Source: CAD feature listing. Evaluate the final solid. Frame: model axes, mm. A direction names the side the tool comes from. Coordinates: 2 decimals unless noted, no trailing zeros. Order: outer loops, then holes, each group sorted by start corner. A loop starts at its lowest first (then second) coordinate and runs counter-clockwise, first axis right, second up.
Autodesk Inventor part; units mm, degrees
ref_plane "YZ Plane" through (0, 0, 0) normal (1, 0, 0) x (0, 1, 0)
ref_plane "XZ Plane" through (0, 0, 0) normal (0, 1, 0) x (-1, 0, 0)
ref_plane "XY Plane" through (0, 0, 0) normal (0, 0, 1) x (1, 0, 0)
sketch "Sketch1" plane through (0, 0, 0) normal (0, 1, 0) x (-1, 0, 0)
  line L0 (10, -14) -> (-10, -14)
  line L1 (-10, -14) -> (-10, 14)
  line L2 (-10, 14) -> (10, 14)
  line L3 (10, 14) -> (10, -14)
  line L4 (10, -14) -> (-10, 14) construction
  line L5 (-10, -14) -> (10, 14) construction
  point P0 (0, 0)
  dimension "d0" = 20
  dimension "d1" = 28
extrude "Extrusion1" add sketch "Sketch1" along normal blind 3
sketch "Sketch2" plane through (0, 0, 0) normal (0, -1, 0) x (1, 0, 0)
  line L0 (-10, 14) -> (10, 14)
  line L1 (-10, 14) -> (10, 14)
  line L2 (10, 14) -> (10, 11)
  line L3 (10, 11) -> (-10, 11)
  line L4 (-10, 11) -> (-10, 14)
  point P0 (0, 0)
  dimension "d4" = 20
  dimension "d5" = 3
extrude "Extrusion2" add sketch "Sketch2" along normal blind 25
sketch "Sketch3" plane through (10, 0, -14) normal (1, 0, 0) x (0, 0, -1)
  line L0 (-25, 0) -> (-25, -25)
  line L1 (0, 0) -> (-25, 0)
  line L2 (0, 0) -> (-25, 0)
  line L3 (-25, 0) -> (-25, -25)
  line L4 (-25, -25) -> (-22, -25)
  line L5 (-22, -25) -> (-22, -22)
  line L6 (0, 0) -> (0, 3)
  line L7 (0, 0) -> (0, -3)
  line L8 (0, -3) -> (-3, -3)
  line L9 (-3, -3) -> (-22, -22)
  point P0 (-14, 0)
  dimension "d8" = 3
  dimension "d9" = 3
  dimension "d10" = 3
  dimension "d11" = 3
extrude "Extrusion3" add sketch "Sketch3" against normal blind 2
mirror "Mirror1" about plane through (0, 0, 0) normal (1, 0, 0) of "Extrusion3"
sketch "Sketch4" plane through (-10, 3, 14) normal (0, 0, 1) x (1, 0, 0)
  line L0 (2, -28) -> (18, -28)
  line L1 (6.75, -9) -> (13.25, -9)
  line L2 (13.25, -9) -> (13.25, -19)
  line L3 (13.25, -19) -> (6.75, -19)
  line L4 (6.75, -19) -> (6.75, -9)
  line L5 (6.75, -9) -> (13.25, -19) construction
  line L6 (13.25, -9) -> (6.75, -19) construction
  arc A0 (13.25, -9) -> (6.75, -9) centre (10, -9) ccw
  arc A1 (6.75, -19) -> (13.25, -19) centre (10, -19) ccw
  point P0 (10, -3)
  point P1 (10, -14)
  dimension "d14" = 6.5
  dimension "d15" = 10
extrude "Extrusion4" cut sketch "Sketch4" against normal through all
sketch "Sketch5" plane through (0, 3, 0) normal (0, 1, 0) x (1, 0, 0)
  line L0 (3.25, -5) -> (-3.25, -5)
  line L1 (-3.25, -5) -> (-3.25, 5)
  line L2 (-3.25, 5) -> (3.25, 5)
  line L3 (3.25, 5) -> (3.25, -5)
  line L4 (3.25, -5) -> (-3.25, 5) construction
  line L5 (-3.25, -5) -> (3.25, 5) construction
  arc A0 (-3.25, -5) -> (3.25, -5) centre (0, -5) ccw
  arc A1 (3.25, 5) -> (-3.25, 5) centre (0, 5) ccw
  point P0 (0, 0)
  dimension "d18" = 6.5
  dimension "d19" = 10
extrude "Extrusion5" cut sketch "Sketch5" against normal through all
properties part number "Ke NHOM 28x28x20"
1. Access query for faces 5 (the face through (0.07, -2.75, 12.52)), 6 (the face through (4, 0, -1)), 7 (the face through (-3.25, 2, 0)), 8 (the face through (-9, -23, 8)). Directions: +Z, -Z, +X, -X, +Y, -Y. A direction counts if a zero-diameter tool reaches every point of the face in a straight line with its end or side. Return the directions, or none.
Findings:
face 5: +Z, -Z
face 6: -Z, -Y
face 7: +Y, -Y
face 8: -Z, +X, -X, -Y
2. Section query D-D on y = -1.25. Return loops of the section in (x, z), plus the area to 3 significant figures.
Findings:
outline: (-10, -14) - (-8, -14) - (-8, 11) - (8, 11) - (8, -14) - (10, -14) - (10, 14) - (-10, 14) - close
area: 160 mm2
3. Section query A-A on y = -10.5. Return loops of the section in (x, z).
Findings:
outline: (-10, -3.5) - (-8, -3.5) - (-8, 11) - (-3.25, 11) - (-3.25, 14) - (-10, 14) - close; (3.25, 11) - (8, 11) - (8, -3.5) - (10, -3.5) - (10, 14) - (3.25, 14) - close
4. Draft query along Z for faces 1 (the face through (-10, -8, 3)), 2 (the face through (-0.07, 1.52, 8.25)), 3 (the face through (-4, -11, 14)), 4 (the face through (9, -12, -2)). Return one class per face: released by +Z, released by -Z, zero draft, split by the parting line, or undercut.
Findings:
face 1: zero draft
face 2: undercut
face 3: released by +Z
face 4: released by -Z
5. Section query B-B on x = 0. Return loops of the section in (y, z), plus the area to 3 significant figures.
Findings:
outline: (-25, 11) - (-19.25, 11) - (-19.25, 14) - (-25, 14) - close; (-2.75, 11) - (0, 11) - (0, 8.25) - (3, 8.25) - (3, 14) - (-2.75, 14) - close; (0, -14) - (3, -14) - (3, -8.25) - (0, -8.25) - close
area: 60.0 mm2
6. Section query C-C on z = 0.75. Return loops of the section in (x, y), plus the area to 3 significant figures.
Findings:
outline: (-10, -14.75) - (-8, -14.75) - (-8, 0) - (-3.25, 0) - (-3.25, 3) - (-10, 3) - close; (3.25, 0) - (8, 0) - (8, -14.75) - (10, -14.75) - (10, 3) - (3.25, 3) - close
area: 99.5 mm2
7. Pin query (flat end, axial travel): P1, Ø2, axis at x = 9, y = -23.5, coming from the -Z side; P2, Ø1.6, axis at x = -9, z = -13, coming from the -Y side; P3, Ø5, axis at y = -6.5, z = -9.5, coming from the +X side; P4, Ø5, axis at x = 3.5, z = -3.5, coming from the -Y side. Return the tip coordinate at first contact, or that it passes through.
Findings:
P1: stops at z = 8
P2: stops at y = -3
P3: stops at x = 10
P4: stops at y = 0
8. Ray query, line 1 (X direction, y = -3, z = -5.75); line 2 (Y direction, x = -8.75, z = -4); line 3 (Y direction, x = 3.5, z = -2.25). Return the intervals inside material, ascending.
Findings:
line 1: x = -10 to -8, 8 to 10
line 2: y = -10 to 3
line 3: y = 0 to 3
